```python
from build123d import *

# Parameters (mm, degrees)
F0_R          = 12.7
F0_R_2        = 9.525
F2_DEPTH      = 6.35
F4_DEPTH      = 25.4
F6_DEPTH      = 2.54
F6_DEPTH_BACK = 2.54
F7_T4_DEPTH   = 24.8484443303
F7_T12_DEPTH  = 24.8484443303
F7_T19_DEPTH  = 5.1569640636
F7_T24_DEPTH  = 5.1569640636
F8_T4_DEPTH   = 24.8484443303
F8_T12_DEPTH  = 24.8484443303
F8_T19_DEPTH  = 5.1569640636
F8_T24_DEPTH  = 5.1569640636


# Not quite as in the source:
# - a fillet or chamfer that OpenCascade refuses, or shapes differently, is made with other operations: its cross-section is extruded or revolved along the edge and cut away or added


with BuildPart() as f2:
    # F0 (on Top) → F2 (new body)
    with BuildSketch(Plane.XY):
        Circle(F0_R)
        Circle(F0_R_2, mode=Mode.SUBTRACT)
    extrude(amount=F2_DEPTH)

    # F3 (on face) → F4 (cut)
    with BuildSketch(Plane.XY.offset(6.35)):
        with BuildLine():
            Line((2.0157811232, 1.8745124225), (-12.0961464615, 3.8695272039))
            ThreePointArc((-12.0961464615, 3.8695272039), (-12.7, 0), (-12.0961464615, -3.8695272039))
            Line((-12.0961464615, -3.8695272039), (2.0157811232, -1.8745124225))
            Line((2.0157811232, -1.8745124225), (2.0157811232, 1.8745124225))
        make_face()
    extrude(amount=-F4_DEPTH, mode=Mode.SUBTRACT)

    # F5 (on Front) → F6 (join, two sides)
    with BuildSketch(Plane.XZ) as f6_sk:
        Polygon((10.5609930441, 5.1569640636), (10.7068819925, 0), (28.8828521035, 0), (15.0134566239, 13.0622601137), (13.0563958547, 13.0622601137), (17.1839392743, 5.1569640636), align=None)
    extrude(amount=F6_DEPTH)
    extrude(f6_sk.sketch, amount=-F6_DEPTH_BACK)

    # F7: fillet of radius 12.7 on 1 edges, made by hand


with BuildPart() as f7_tool2:
    # F7_s3 → F7_t4 (new body)
    with BuildSketch(Plane.XY.offset(24.8484443303)):
        with BuildLine():
            ThreePointArc((10.16, -7.62), (14.6403873372, -3.8807746743), (20.32, -2.54))
            Line((20.32, -2.54), (12.4434078933, -2.54))
            ThreePointArc((12.4434078933, -2.54), (11.5836139481, -5.206715654), (10.16, -7.62))
        make_face()
    extrude(amount=-F7_T4_DEPTH)

    split(bisect_by=Plane.XY.offset(6.35), keep=Keep.TOP)

    split(bisect_by=Plane(origin=(15.6186590558, 0, 8.1548740238), x_dir=(0, 1, 0), z_dir=(0.8864449555, 0, 0.4628340317)), keep=Keep.TOP)

    split(bisect_by=Plane.XY.offset(13.0622601137), keep=Keep.BOTTOM)

    split(bisect_by=Plane(origin=(13.5765905704, 0, 14.4155071364), x_dir=(0, 1, 0), z_dir=(-0.6856071252, 0, -0.7279717507)), keep=Keep.TOP)


with BuildPart() as f2_1:
    add(f2.part)

    # F7_t1: union F7_tool2
    add(f7_tool2.part)


with BuildPart() as f7_tool10:
    # F7_s11 → F7_t12 (new body)
    with BuildSketch(Plane.XY.offset(24.8484443303)):
        with BuildLine():
            ThreePointArc((10.16, -7.62), (14.6403873372, -3.8807746743), (20.32, -2.54))
            Line((20.32, -2.54), (12.4434078933, -2.54))
            ThreePointArc((12.4434078933, -2.54), (11.5836139481, -5.206715654), (10.16, -7.62))
        make_face()
    extrude(amount=-F7_T12_DEPTH)

    split(bisect_by=Plane.XY.offset(5.1569640636), keep=Keep.TOP)

    split(bisect_by=Plane.XY.offset(6.35), keep=Keep.BOTTOM)

    split(bisect_by=Plane(origin=(15.6186590558, 0, 8.1548740238), x_dir=(0, 1, 0), z_dir=(0.8864449555, 0, 0.4628340317)), keep=Keep.TOP)


with BuildPart() as f2_2:
    add(f2_1.part)

    # F7_t9: union F7_tool10
    add(f7_tool10.part)


with BuildPart() as f7_tool17:
    # F7_s18 → F7_t19 (new body)
    with BuildSketch(Plane.XY.offset(5.1569640636)):
        with BuildLine():
            ThreePointArc((10.16, -7.62), (14.6403873372, -3.8807746743), (20.32, -2.54))
            Line((20.32, -2.54), (12.4434078933, -2.54))
            ThreePointArc((12.4434078933, -2.54), (11.5836139481, -5.206715654), (10.16, -7.62))
        make_face()
    extrude(amount=-F7_T19_DEPTH)

    split(bisect_by=Plane(origin=(15.6186590558, 0, 8.1548740238), x_dir=(0, 1, 0), z_dir=(0.8864449555, 0, 0.4628340317)), keep=Keep.TOP)


with BuildPart() as f2_3:
    add(f2_2.part)

    # F7_t16: union F7_tool17
    add(f7_tool17.part)


with BuildPart() as f7_tool22:
    # F7_s23 → F7_t24 (new body)
    with BuildSketch(Plane.XY.offset(5.1569640636)):
        with BuildLine():
            ThreePointArc((10.16, -7.62), (14.6403873372, -3.8807746743), (20.32, -2.54))
            Line((20.32, -2.54), (12.4434078933, -2.54))
            ThreePointArc((12.4434078933, -2.54), (11.5836139481, -5.206715654), (10.16, -7.62))
        make_face()
    extrude(amount=-F7_T24_DEPTH)

    split(bisect_by=Plane(origin=(15.6186590558, 0, 8.1548740238), x_dir=(0, 1, 0), z_dir=(-0.8864449555, 0, -0.4628340317)), keep=Keep.TOP)


with BuildPart() as f2_4:
    add(f2_3.part)

    # F7_t21: union F7_tool22
    add(f7_tool22.part)

    # F8: fillet of radius 12.7 on 1 edges, made by hand


with BuildPart() as f8_tool2:
    # F8_s3 → F8_t4 (new body)
    with BuildSketch(Plane.XY.offset(24.8484443303)):
        with BuildLine():
            ThreePointArc((10.16, 7.62), (14.6403873372, 3.8807746743), (20.32, 2.54))
            Line((20.32, 2.54), (12.4434078933, 2.54))
            ThreePointArc((12.4434078933, 2.54), (11.5836139481, 5.206715654), (10.16, 7.62))
        make_face()
    extrude(amount=-F8_T4_DEPTH)

    split(bisect_by=Plane.XY.offset(6.35), keep=Keep.TOP)

    split(bisect_by=Plane(origin=(15.6186590558, 0, 8.1548740238), x_dir=(0, 1, 0), z_dir=(0.8864449555, 0, 0.4628340317)), keep=Keep.TOP)

    split(bisect_by=Plane.XY.offset(13.0622601137), keep=Keep.BOTTOM)

    split(bisect_by=Plane(origin=(13.5765905704, 0, 14.4155071364), x_dir=(0, 1, 0), z_dir=(-0.6856071252, 0, -0.7279717507)), keep=Keep.TOP)


with BuildPart() as f2_5:
    add(f2_4.part)

    # F8_t1: union F8_tool2
    add(f8_tool2.part)


with BuildPart() as f8_tool10:
    # F8_s11 → F8_t12 (new body)
    with BuildSketch(Plane.XY.offset(24.8484443303)):
        with BuildLine():
            ThreePointArc((10.16, 7.62), (14.6403873372, 3.8807746743), (20.32, 2.54))
            Line((20.32, 2.54), (12.4434078933, 2.54))
            ThreePointArc((12.4434078933, 2.54), (11.5836139481, 5.206715654), (10.16, 7.62))
        make_face()
    extrude(amount=-F8_T12_DEPTH)

    split(bisect_by=Plane.XY.offset(5.1569640636), keep=Keep.TOP)

    split(bisect_by=Plane.XY.offset(6.35), keep=Keep.BOTTOM)

    split(bisect_by=Plane(origin=(15.6186590558, 0, 8.1548740238), x_dir=(0, 1, 0), z_dir=(0.8864449555, 0, 0.4628340317)), keep=Keep.TOP)


with BuildPart() as f2_6:
    add(f2_5.part)

    # F8_t9: union F8_tool10
    add(f8_tool10.part)


with BuildPart() as f8_tool17:
    # F8_s18 → F8_t19 (new body)
    with BuildSketch(Plane.XY.offset(5.1569640636)):
        with BuildLine():
            ThreePointArc((10.16, 7.62), (14.6403873372, 3.8807746743), (20.32, 2.54))
            Line((20.32, 2.54), (12.4434078933, 2.54))
            ThreePointArc((12.4434078933, 2.54), (11.5836139481, 5.206715654), (10.16, 7.62))
        make_face()
    extrude(amount=-F8_T19_DEPTH)

    split(bisect_by=Plane(origin=(15.6186590558, 0, 8.1548740238), x_dir=(0, 1, 0), z_dir=(0.8864449555, 0, 0.4628340317)), keep=Keep.TOP)


with BuildPart() as f2_7:
    add(f2_6.part)

    # F8_t16: union F8_tool17
    add(f8_tool17.part)


with BuildPart() as f8_tool22:
    # F8_s23 → F8_t24 (new body)
    with BuildSketch(Plane.XY.offset(5.1569640636)):
        with BuildLine():
            ThreePointArc((10.16, 7.62), (14.6403873372, 3.8807746743), (20.32, 2.54))
            Line((20.32, 2.54), (12.4434078933, 2.54))
            ThreePointArc((12.4434078933, 2.54), (11.5836139481, 5.206715654), (10.16, 7.62))
        make_face()
    extrude(amount=-F8_T24_DEPTH)

    split(bisect_by=Plane(origin=(15.6186590558, 0, 8.1548740238), x_dir=(0, 1, 0), z_dir=(-0.8864449555, 0, -0.4628340317)), keep=Keep.TOP)


with BuildPart() as f2_8:
    add(f2_7.part)

    # F8_t21: union F8_tool22
    add(f8_tool22.part)


solid = f2_8.part
```
Part model, mm, in its own coordinate system. A direction names the side the tool comes from. Coordinates: 2 decimals unless noted, no trailing zeros. Order: outer loops, then holes, each group sorted by start corner. A loop starts at its lowest first (then second) coordinate and runs counter-clockwise, first axis right, second up. Notation, with made-up numbers: (42, -10.75) - (92, -10.75) arc R26 cw to (92, 19.25) - close; hole circle Ø8 at (55.25, -14.5). An arc over 180 degrees is marked (long way). Return JSON: item names as keys, results as strings. Group by question number.
Item 1: Which spindle directions (+Z, -Z, +X, -X, +Y, -Y) get a long thin tool onto all of the face, cutting with end or side? Do faces 5 (the face through (23, -2.54, 2)), 6 (the face through (9.518, -0.37, 3.131)), 7 (the face through (-10.47, 3.64, 3.22)). Say none if no direction does.
Item 2: Cut at C-C (y = -8.75). List the corners of the cut face in (x, z), plus the area to 3 significant figures.
Item 3: Cut at B-B (y = 0). List the corners of the cut face in (x, z) (3 decimals), plus the area to 3 significant figures.
Item 4: Pin check, flat tips, straight feed: pin 1 (4 mm diameter, centred on x = 18, z = 5, fed in from -Y); pin 2 (4 mm diameter, centred on x = 1, y = -9, fed in from +Z); pin 3 (4 mm diameter, centred on x = 26.5, z = 2.5, fed in from +Y). Stop position of each tip, or through.
Item 5: Cut at D-D (z = 11.75). List the corners of the cut face in (x, y).
Item 6: Drill centre lines: probe 1 along Y at (x, z) = (0, 2.25) (3 decimals); probe 2 along X at (y, z) = (-7.75, 2.5); probe 3 along X at (y, z) = (8.5, 6). Where is each one in solid material? Low to high. Write a range as from..to.
Item 7: Pull direction Z, two halves, no side cores. Call faces 1 (the face through (9, -5, 6.35)), 2 (the face through (23, 2.54, 2)), 3 (the face through (14, 0, 5.157)), 4 (the face through (10, 1, 0)): pulls with the +Z half, pulls with the -Z half, needs draft (parallel to the pull), parting line crosses it, or undercut.
Item 8: Cut at A-A (x = -3). List the corners of the cut face in (y, z), plus the area to 3 significant figures.
Check values:
{
 "1": {"face 5": "+Z, -Z, +X, -Y", "face 6": "+Z, -Z", "face 7": "+Z, -Z, -X"},
 "2": {"outline": "(-9.2, 0) - (-3.76, 0) - (-3.76, 6.35) - (-9.2, 6.35) - close; (3.76, 0) - (9.2, 0) - (9.2, 6.35) - (3.76, 6.35) - close", "area": "69.1 mm2"},
 "3": {"outline": "(9.525, 0) - (28.883, 0) - (15.013, 13.062) - (13.056, 13.062) - (17.184, 5.157) - (12.7, 5.157) - (12.7, 6.35) - (9.525, 6.35) - close", "area": "122 mm2"},
 "4": {"pin 1": "stops at y = -3.3", "pin 2": "stops at z = 6.35", "pin 3": "stops at y = 2.54"},
 "5": {"outline": "(13.74, -4.38) arc R12.7 cw to (16.41, -3.16) - (16.41, 3.16) arc R12.7 cw to (13.74, 4.38) - close"},
 "6": {"probe 1": "y = -12.7..-9.525, 9.525..12.7", "probe 2": "x = -10.06..-5.54, 5.54..10.06", "probe 3": "x = -9.44..-4.3, 4.3..9.44"},
 "7": {"face 1": "pulls with the +Z half", "face 2": "needs draft", "face 3": "undercut", "face 4": "pulls with the -Z half"},
 "8": {"outline": "(-12.34, 0) - (-9.04, 0) - (-9.04, 6.35) - (-12.34, 6.35) - close; (9.04, 0) - (12.34, 0) - (12.34, 6.35) - (9.04, 6.35) - close", "area": "41.9 mm2"}
}
